```python
from build123d import *

# Parameters (mm, degrees)
F2_R = 2.53999


# Not quite as in the source:
# - a fillet or chamfer is up to 0.001 mm smaller than in the source, because OpenCascade refuses the exact size


with BuildPart() as f1:
    # F0 (on Front) → F1 (revolve)
    with BuildSketch(Plane.XZ):
        Polygon((-123.19, 0), (0, 0), (0, 3.81), (-107.95, 3.81), (-107.95, 20.32), (-104.14, 20.32), (-104.14, 25.4), (-127, 25.4), (-127, 20.32), (-123.19, 20.32), align=None)
    revolve(axis=Axis((0, 0, 1.905), (0, 0, -1)))

    # F2 (radius 2.54 in the source; OpenCascade refuses exactly that, so slightly less here)
    f2_edges = [f1.edges().sort_by_distance(p)[0] for p in [
        (127, 0, 25.4),
        (127, 0, 20.32),
        (-127, 0, 22.86),
        (104.14, 0, 20.32),
        (104.14, 0, 25.4),
        (-104.14, 0, 22.86),
    ]]
    fillet(f2_edges, radius=F2_R)


solid = f1.part
```
Check sheet for the modelled part. Datum: model origin and axes. Units: mm. A direction names the side the tool comes from. Round coordinates to 2 decimals unless told otherwise and drop trailing zeros. Loops run counter-clockwise (first coordinate to the right, second up) from the corner with the lowest first, then second, coordinate; pieces in that order, holes last. Notation, with made-up numbers: (-22.75, -19.75) - (16.25, -19.75) arc R20 cw to (16.25, -11.75) - close; hole circle Ø10 at (-23, 50.5). An arc over 180 degrees is marked (long way). Write item = value, one per line. Start each with the question number.
Q1. Depth check by flat-ended pin: P1, Ø10, axis at x = -47.5, y = 85.5, coming from the +Z side; P2, Ø4, axis at y = 22.5, z = 18, coming from the -X side; P3, Ø6, axis at x = -41.5, z = 20, coming from the -Y side. Enter the tip coordinate at first touch or a pass-through.
Q2. Section check C-C (z = 8.75). Record the boundary of the cut face in (x, y), plus the area to 3 significant figures.
Q3. Release check for a two-part mould opening along Z. For faces 1 (the face through (92, 56, 25.4)), 2 (the face through (79.56, 72.96, 12.18)), 3 (the face through (26.71, -120.26, 10.02)) record: pulls with the +Z half, pulls with the -Z half, needs draft (parallel to the pull), parting line crosses it, or undercut.
Q4. Thickness scan on L1, parallel to Y at x = 0, z = 22.95; L2, parallel to Y at x = 0, z = 13.75; L3, parallel to Z at x = 1, y = -13. Record the ranges inside material, lowest first.
Q5. Access from +Z, -Z, +X, -X, +Y, -Y to the whole of each face (thin tool, end or side, straight path). Record for faces 4 (the face through (120.4, 28.2, 20.32)), 5 (the face through (2, 2, 0)), 6 (the face through (104.5, 24.5, 20.32)).
Derived:
q1.P1 = 3.81
q1.P2 = -121.47
q1.P3 = -120.63
q2.outline = circle Ø246.38 at (0, 0); hole circle Ø215.9 at (0, 0)
q2.area = 11,100 mm^2
q3.face_1 = pulls with the +Z half
q3.face_2 = undercut
q3.face_3 = needs draft
q4.L1 = -127 to -104.14, 104.14 to 127
q4.L2 = -123.19 to -107.95, 107.95 to 123.19
q4.L3 = 0 to 3.81
q5.face_4 = -Z
q5.face_5 = -Z, +X, -X, +Y, -Y
q5.face_6 = none
